Source: CAD feature listing. Evaluate the final solid. Frame: model axes, mm. A direction names the side the tool comes from. Give positions to 0.01 mm unless a question says otherwise; leave off trailing zeros. Order: outer loops, then holes, each group sorted by start corner. A loop starts at its lowest first (then second) coordinate and runs counter-clockwise, first axis right, second up.
1) Section B-B, the plane x = 6.25. Return loops of the section in (y, z), plus the area to 3 significant figures.
2) Access query for faces 1 (the face through (0, -5, 0)), 2 (the face through (5.18, -5.16, 20.28)), 3 (the face through (-5.996, -5.009, 10.574)). Directions: +Z, -Z, +X, -X, +Y, -Y. A direction counts if a zero-diameter tool reaches every point of the face in a straight line with its end or side. Return the directions, or none.
3) Section D-D, the plane z = 8.75. Return loops of the section in (x, y), plus the area to 3 significant figures.
4) Section C-C, the plane y = -8.75. Return loops of the section in (x, z).
5) Draft query along X for faces 4 (the face through (-7.81, -5.01, 12.4)), 5 (the face through (-5.075, -5.004, 20.492)), 6 (the face through (7.886, -5.009, 12.057)), 7 (the face through (-7, 0, 10)). Return one class per face: released by +X, released by -X, zero draft, split by the parting line, or undercut.
6) Section A-A, the plane z = 18.75. Return loops of the section in (x, y), plus the area to 3 significant figures.
7) Material intervals for line 1 (Z direction, x = 3.5, y = -1.75); line 2 (X direction, y = -5.5, z = 18.25); line 3 (X direction, y = -7.5, z = 21), sorted ascending.
8) First-contact query: P1, Ø1, axis at x = 2, y = -6, coming from the +Z side; P2, Ø1.5, axis at y = -8, z = 14.5, coming from the -X side; P3, Ø1, axis at x = 0.5, y = -2, coming from the -Z side. Flat tips, straight axial feed; report the tip coordinate or a pass-through.
```python
from build123d import *

# Parameters (mm, degrees)
F1_DEPTH = 10.16
F3_DEPTH = 20.32
F5_DEPTH = 20.32


with BuildPart() as f1:
    # F0 (on Front) → F1 (new body)
    with BuildSketch(Plane.XZ):
        Polygon((-10.16, 0), (0, 0), (10.149805, 0), (5.557302, 24.457385), (3.397579, 24.457385), (7.615184, 1.996521), (0, 1.996521), (-7.62, 1.996521), (-3.366859, 24.457385), (-5.528802, 24.457385), align=None)
    extrude(amount=F1_DEPTH)

    # F2 (on face) → F3 (cut)
    with BuildSketch(Plane.XY.offset(24.457385)):
        with BuildLine():
            Line((-3.366859, -10.16), (-3.366859, 0))
            ThreePointArc((-3.366859, 0), (-5.074936, -5.08), (-3.366859, -10.16))
        make_face()
    extrude(amount=-F3_DEPTH, mode=Mode.SUBTRACT)

    # F4 (on face) → F5 (cut)
    with BuildSketch(Plane.XY.offset(24.457385)):
        with BuildLine():
            Line((3.397579, 0), (3.397579, -10.16))
            ThreePointArc((3.397579, -10.16), (5.178992, -5.08), (3.397579, 0))
        make_face()
    extrude(amount=-F5_DEPTH, mode=Mode.SUBTRACT)


solid = f1.part
```
From the geometry:
1. outline: (-10.16, 0) - (0, 0) - (0, 2) - (-10.16, 2) - close; (-10.16, 9.27) - (0, 9.27) - (0, 20.77) - (-10.16, 20.77) - close
1. area: 137 mm2
2. face 1: -Z, +X, -X, +Y, -Y
2. face 2: +Z
2. face 3: +Y, -Y
3. outline: (-8.5, -10.16) - (-6.34, -10.16) - (-6.34, 0) - (-8.5, 0) - close; (6.35, -10.16) - (8.51, -10.16) - (8.51, 0) - (6.35, 0) - close
3. area: 43.9 mm2
4. outline: (-10.16, 0) - (10.15, 0) - (5.56, 24.46) - (4.3, 24.46) - (4.3, 19.63) - (7.62, 2) - (-7.62, 2) - (-4.23, 19.89) - (-4.23, 24.46) - (-5.53, 24.46) - close
5. face 4: released by -X
5. face 5: undercut
5. face 6: released by +X
5. face 7: zero draft
6. outline: (-6.61, -10.16) - (-4.45, -10.16) - (-4.45, -8.27) arc R8.41 cw to (-4.45, -1.89) - (-4.45, 0) - (-6.61, 0) - close; (4.47, -10.16) - (6.63, -10.16) - (6.63, 0) - (4.47, 0) - (4.47, -1.76) arc R8.13 cw to (4.47, -8.4) - close
6. area: 38.0 mm2
7. line 1: z = 0 to 2
7. line 2: x = -6.7 to -5.06, 5.17 to 6.72
7. line 3: x = -6.18 to -4.72, 4.81 to 6.21
8. P1: stops at z = 2
8. P2: stops at x = -7.56
8. P3: stops at z = 0
